CAD build for the part. Positions are in the model's coordinates, mm. Coordinates: 2 decimals unless noted, no trailing zeros. Loops run counter-clockwise (first coordinate to the right, second up) from the corner with the lowest first, then second, coordinate; pieces in that order, holes last. Notation, with made-up numbers: (22, 50) -> (53, 50) arc R22 ccw to (53, 77) -> close; hole circle Ø7 at (-10.75, -6.5). An arc over 180 degrees is marked (long way). Write item = value, one per line. Start each with the question number.
(1) Band-saw the part on B-B (x = -13). Write the cut outline in (y, z).
(2) Flat gauge pin, fed straight in: P1, Ø3.5, axis at x = 0, z = 0, coming from the -Y side. Where does the tip first touch, or does it go through?
(3) Band-saw the part on A-A (y = 0.6). Write the cut outline in (x, z), and give its area (3 significant figures).
(4) Band-saw the part on C-C (z = -31.75). Write the cut outline in (x, y), and give its area (3 significant figures).
(5) Pull direction Z, two halves, no side cores. Call faces 1 (the face through (-11.195, 0.783, -50.619)), 2 (the face through (-24.926, 0.783, -29.618)), 3 (the face through (-17.84, 0.783, -12.125)): +Z half, -Z half, draft (parallel to the pull), parting line (faces both ways), or undercut.
(6) Drill centre lines: line 1 (Z direction, x = -25.5, y = 1.35); line 2 (Z direction, x = -25.4, y = 0.8); line 3 (Z direction, x = -9, y = 0.2). Where is each one in solid material? Low to high. Write a range as from..to.
(7) Band-saw the part on D-D (z = -5.5). Write the cut outline in (x, y), and give its area (3 significant figures).
Autodesk Inventor part; units mm, degrees
ref_plane "YZ Plane" through (0, 0, 0) normal (1, 0, 0) x (0, 1, 0)
ref_plane "XZ Plane" through (0, 0, 0) normal (0, 1, 0) x (-1, 0, 0)
ref_plane "XY Plane" through (0, 0, 0) normal (0, 0, 1) x (1, 0, 0)
sketch "main" plane through (0, 0, 0) normal (0, 0, 1) x (1, 0, 0)
  circle A0 centre (7.7194, -42.2476) radius 2.1844
  circle A1 centre (20.4194, -29.5476) radius 2.1844
  circle A2 centre (-4.9806, 2.2024) radius 2.0955
  arc A3 (-0.0233, 6.1707) -> (-11.0863, 0.4579) centre (-4.9806, 2.2024) ccw
  arc A4 (1.6137, -43.9921) -> (12.2065, -46.7408) centre (7.7194, -42.2476) ccw
  arc A5 (24.9151, -34.0494) -> (25.3862, -25.5717) centre (20.4194, -29.5476) ccw
  line L0 (12.2065, -46.7408) -> (24.9151, -34.0494)
  line L1 (1.6137, -43.9921) -> (-11.0863, 0.4579)
  line L2 (25.3862, -25.5717) -> (-0.0233, 6.1707)
  point P0 (8.3889, -23.6516)
  dimension "d0" = 12.7
  dimension "d1" = 12.7
sketch "Sketch1" plane through (0, 0, 0) normal (0, 1, 0) x (-1, 0, 0)
  circle A0 centre (12.7, -44.45) radius 2.1844
  circle A1 centre (25.4, -31.75) radius 2.1844
  circle A2 centre (0, 0) radius 2.0955
  arc A3 (4.9573, 3.9683) -> (-6.1057, -1.7445) centre (0, 0) ccw
  arc A4 (6.5943, -46.1945) -> (17.1871, -48.9432) centre (12.7, -44.45) ccw
  arc A5 (29.8957, -36.2518) -> (30.3668, -27.7741) centre (25.4, -31.75) ccw
  line L0 (17.1871, -48.9432) -> (29.8957, -36.2518)
  line L1 (6.5943, -46.1945) -> (-6.1057, -1.7445)
  line L2 (30.3668, -27.7741) -> (4.9573, 3.9683)
extrude "Extrusion1" add sketch "Sketch1" along normal blind 1.5875
properties part number "gusset" material "Acetal Resin, White"
Findings below:
q1.outline = (0, -50.79) -> (1.59, -50.79) -> (1.59, -46.61) -> (0, -46.61) -> close; (0, -42.29) -> (1.59, -42.29) -> (1.59, -6.08) -> (0, -6.08) -> close
q2.P1 = through
q3.outline = (-30.37, -27.77) arc R6.36 ccw to (-29.9, -36.25) -> (-17.19, -48.94) arc R6.35 ccw to (-6.59, -46.19) -> (6.11, -1.74) arc R6.35 ccw to (-4.96, 3.97) -> close; hole circle Ø4.37 at (-25.4, -31.75); hole circle Ø4.37 at (-12.7, -44.45); hole circle Ø4.19 at (0, 0)
q3.area = 1,110 mm²
q4.outline = (-31.76, 0) -> (-27.58, 0) -> (-27.58, 1.59) -> (-31.76, 1.59) -> close; (-23.22, 0) -> (-2.47, 0) -> (-2.47, 1.59) -> (-23.22, 1.59) -> close
q4.area = 39.6 mm²
q5.face_1 = -Z half
q5.face_2 = undercut
q5.face_3 = +Z half
q6.line_1 = -40.64..-33.93, -29.57..-21.69
q6.line_2 = -40.74..-33.93, -29.57..-21.57
q6.line_3 = -49.61..-1.08
q7.outline = (-12.54, 0) -> (5.03, 0) -> (5.03, 1.59) -> (-12.54, 1.59) -> close
q7.area = 27.9 mm²
